Source: three-view drawing plus pictorial views. Frame: mm from the lowest corner of the part. Round coordinates to 2 decimals unless told otherwise and drop trailing zeros. Write each loop counter-clockwise with the first axis right and the second up, starting at its lowest first coordinate (ties: lowest second). Pieces come first, ordered by that corner, then holes. Notation, with made-up numbers: M -24.75,46.5 L 14.25,46.5 A4 cw 14.25,53.5 Z; hole C 66,27 d6. An arc over 180 degrees is marked long. Answer in a Markdown table with one row per item.
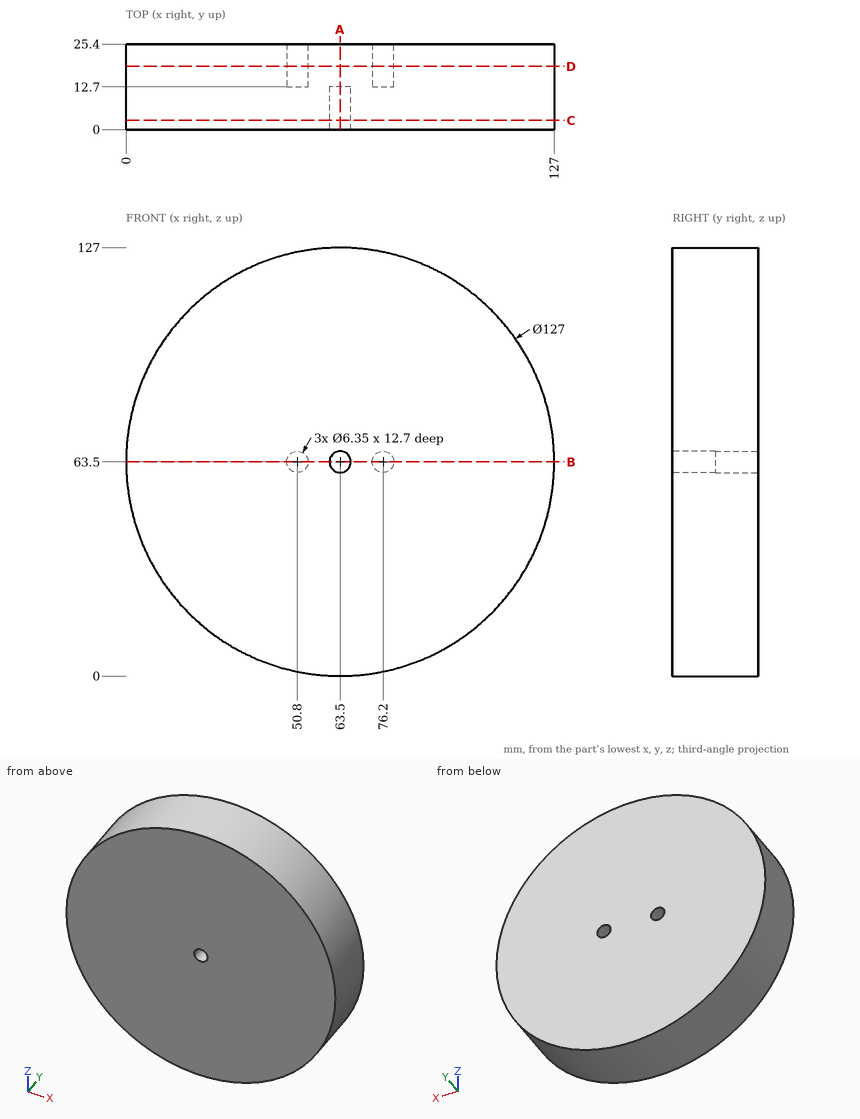
Q1. Contact query for flat-ended pins moving along their axis: pin 1 Ø1 at (y, z) = (8.5, 99) entering from -X; pin 2 Ø1.5 at (x, y) = (71.5, 8.5) entering from -Z; pin 3 Ø4 at (y, z) = (22.5, 85.5) entering from +X. Output: stop coordinate, or through.
Solutions:
| item | result |
|---|---|
| pin 1 | stops at x = 10.52 |
| pin 2 | stops at z = 0.42 |
| pin 3 | stops at x = 123.77 |
Q2. Section C-C (y = 2.75). Return loops of the section in (x, z) (3 decimals), and give its area (3 significant figures).
Solutions:
| item | result |
|---|---|
| outline | C 63.5,63.5 d127; hole C 63.5,63.5 d6.35 |
| area | 12,600 mm2 |
Q3. Material intervals for probe 1 along X at (y, z) = (22.25, 65); probe 2 along Z at (x, y) = (63.5, 6.25) (3 decimals); probe 3 along Z at (x, y) = (76.2, 20) (3 decimals), sorted ascending.
Solutions:
| item | result |
|---|---|
| probe 1 | x = 0.02 to 48, 53.6 to 73.4, 79 to 126.98 |
| probe 2 | z = 0 to 60.325, 66.675 to 127 |
| probe 3 | z = 1.283 to 60.325, 66.675 to 125.717 |
Q4. Section D-D (y = 18.75). Return loops of the section in (x, z) (3 decimals).
Solutions:
| item | result |
|---|---|
| outline | C 63.5,63.5 d127; hole C 50.8,63.5 d6.35; hole C 76.2,63.5 d6.35 |
Q5. Section B-B (z = 63.5). Return loops of the section in (x, y) (3 decimals).
Solutions:
| item | result |
|---|---|
| outline | M 0,0 L 60.325,0 L 60.325,12.7 L 66.675,12.7 L 66.675,0 L 127,0 L 127,25.4 L 79.375,25.4 L 79.375,12.7 L 73.025,12.7 L 73.025,25.4 L 53.975,25.4 L 53.975,12.7 L 47.625,12.7 L 47.625,25.4 L 0,25.4 Z |
Q6. Section A-A (x = 63.5). Return loops of the section in (y, z) (3 decimals), and give its area (3 significant figures).
Solutions:
| item | result |
|---|---|
| outline | M 0,0 L 25.4,0 L 25.4,127 L 0,127 L 0,66.675 L 12.7,66.675 L 12.7,60.325 L 0,60.325 Z |
| area | 3,150 mm2 |
